```python
from build123d import *

# Parameters (mm, degrees)
SKETCH2_W           = 10
SKETCH2_H           = 79
SKETCH2_R           = 2.5
BOSS_EXTRUDE1_DEPTH = 10
SKETCH3_R           = 2.5
CUT_EXTRUDE1_DEPTH  = 5


with BuildPart() as part:
    # Sketch2 → Boss-Extrude1 (new body)
    with BuildSketch(Plane(origin=(0, 0, 0), x_dir=(0, 0, -1), z_dir=(1, 0, 0))):
        Rectangle(SKETCH2_W, SKETCH2_H)
        with Locations((0, -34.5)):
            Circle(SKETCH2_R, mode=Mode.SUBTRACT)
    extrude(amount=BOSS_EXTRUDE1_DEPTH)

    # Sketch3 → Cut-Extrude1 (cut)
    with BuildSketch(Plane(origin=(0, 39.5, 0), x_dir=(1, 0, 0), z_dir=(0, 1, 0))):
        with Locations((5, 0)):
            Circle(SKETCH3_R)
    extrude(amount=-CUT_EXTRUDE1_DEPTH, mode=Mode.SUBTRACT)


solid = part.part
```
Verification items for the finished model (mm, model axes). A direction names the side the tool comes from. Give positions to 0.01 mm unless a question says otherwise; leave off trailing zeros. Order: outer loops, then holes, each group sorted by start corner. A loop starts at its lowest first (then second) coordinate and runs counter-clockwise, first axis right, second up. Notation, with made-up numbers: (79.25, -9) -> (109.25, -9) arc R32 ccw to (109.25, 17) -> close; hole circle Ø6 at (19, -9.5). An arc over 180 degrees is marked (long way). One line per item, written item: value.
(1) Gauge pin test, flat end, axial feed: pin 1 (3 mm diameter, centred on x = 5, z = 0, fed in from +Y). Record the tip position at first contact, or that the pin passes through.
Final values:
pin 1: y = 34.5
(2) Sectioned sample at D-D on x = 8.75. Record the cut outline in (y, z).
Final values:
outline: (-39.5, -5) -> (39.5, -5) -> (39.5, 5) -> (-39.5, 5) -> close; hole circle Ø5 at (-34.5, 0)
(3) Sectioned sample at A-A on y = -34.5. Record the cut outline in (x, z).
Final values:
outline: (0, -5) -> (10, -5) -> (10, -2.5) -> (0, -2.5) -> close; (0, 2.5) -> (10, 2.5) -> (10, 5) -> (0, 5) -> close
(4) Sectioned sample at B-B on z = 0. Record the cut outline in (x, y), then the cut area to 3 significant figures.
Final values:
outline: (0, -39.5) -> (10, -39.5) -> (10, -37) -> (0, -37) -> close; (0, -32) -> (10, -32) -> (10, 39.5) -> (7.5, 39.5) -> (7.5, 34.5) -> (2.5, 34.5) -> (2.5, 39.5) -> (0, 39.5) -> close
area: 715 mm^2
(5) Scan lines: line 1 along Y through (x, z) = (3.5, 0); line 2 along Z through (x, y) = (5, 37.25); line 3 along Y through (x, z) = (8, 0). Record each from-to range of solid material in increasing order. Write a range as [from, to].
Final values:
line 1: [-39.5, -37], [-32, 34.5]
line 2: [-5, -2.5], [2.5, 5]
line 3: [-39.5, -37], [-32, 39.5]
(6) Sectioned sample at C-C on x = 5. Record the cut outline in (y, z).
Final values:
outline: (-39.5, -5) -> (39.5, -5) -> (39.5, -2.5) -> (34.5, -2.5) -> (34.5, 2.5) -> (39.5, 2.5) -> (39.5, 5) -> (-39.5, 5) -> close; hole circle Ø5 at (-34.5, 0)
(7) Tool access check on faces 1 (the face through (4.93, -32.39, -1.34)), 2 (the face through (5, 34.5, 0)). Record the directions out of +Z, -Z, +X, -X, +Y, -Y that give a thin tool (end or side, any length) a straight path to the whole face; none if there is none.
Final values:
face 1: +X, -X
face 2: +Y
(8) Draft check along Z on faces 3 (the face through (3, 39.5, 2)), 4 (the face through (7.385, 37.035, -0.751)), 5 (the face through (5, -1, -5)). Enter one of: pulls with the +Z half, pulls with the -Z half, needs draft (parallel to the pull), parting line crosses it, or undercut.
Final values:
face 3: needs draft
face 4: undercut
face 5: pulls with the -Z half
